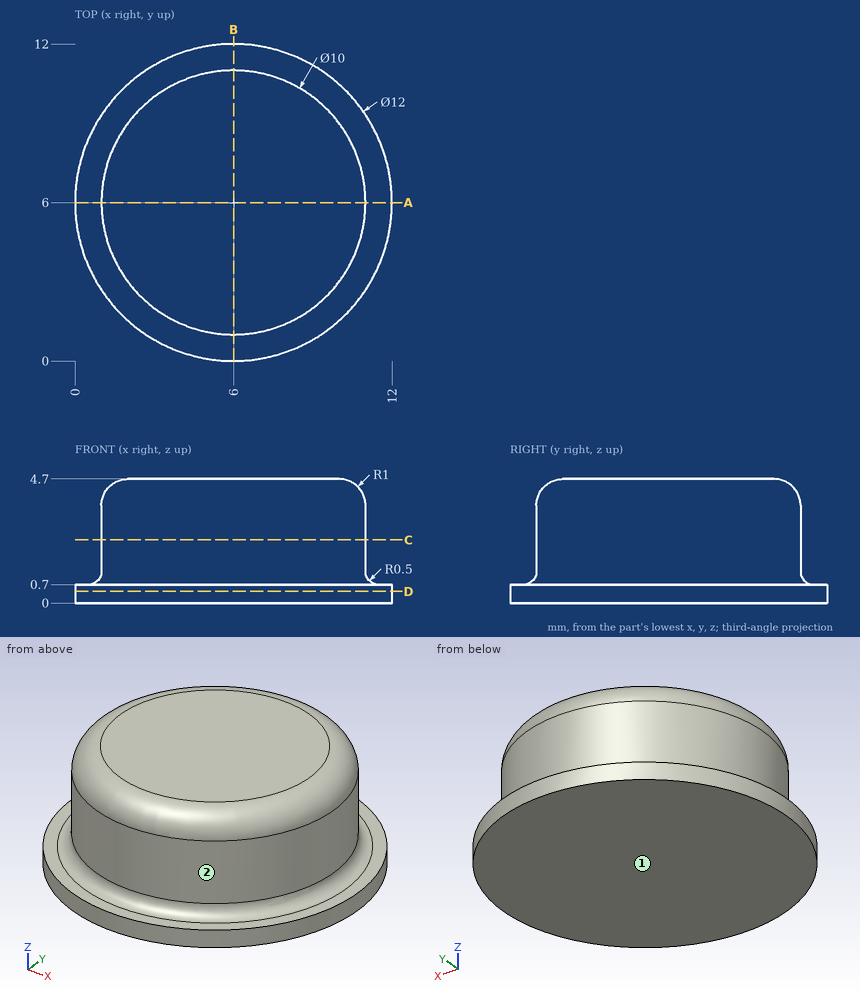
Source: three-view drawing plus pictorial views. Frame: mm from the lowest corner of the part. A direction names the side the tool comes from. Give positions to 0.01 mm unless a question says otherwise; leave off trailing zeros. Loops run counter-clockwise (first coordinate to the right, second up) from the corner with the lowest first, then second, coordinate; pieces in that order, holes last. Notation, with made-up numbers: (-19.75, 77) -> (6.25, 77) arc R17 cw to (6.25, 109) -> close; hole circle Ø10 at (77.25, -7.5). An arc over 180 degrees is marked (long way). Put each result on its own line as item: value. Start each with the question number.
1) Contact query for flat-ended pins moving along their axis: P1, Ø1, axis at x = 5.5, z = 4, coming from the -Y side; P2, Ø2, axis at x = 2, z = 2, coming from the +Y side. Output: stop coordinate, or through.
2) Cut plane A-A (y = 6). Return loops of the section in (x, z), then the cut area to 3 significant figures.
3) Reachability of the marked faces 1 and 2 from +Z, -Z, +X, -X, +Y, -Y: full face, straight path, thin tool, end or side. Return the list, or none.
4) Material intervals for probe 1 along Z at (x, y) = (10, 10.25); probe 2 along X at (y, z) = (3, 2.6); probe 3 along Y at (x, z) = (6, 2.05), sorted ascending.
5) Cut plane D-D (z = 0.45). Return loops of the section in (x, y), then the cut area to 3 significant figures.
6) Cut plane C-C (z = 2.4). Return loops of the section in (x, y), then the cut area to 3 significant figures.
Results are:
1. P1: stops at y = 1
1. P2: stops at y = 10
2. outline: (0, 0) -> (12, 0) -> (12, 0.7) -> (11.5, 0.7) arc R0.5 cw to (11, 1.2) -> (11, 3.7) arc R1 ccw to (10, 4.7) -> (2, 4.7) arc R1 ccw to (1, 3.7) -> (1, 1.2) arc R0.5 cw to (0.5, 0.7) -> (0, 0.7) -> close
2. area: 48.1 mm2
3. face 1: -Z, +X, -X, +Y, -Y
3. face 2: +Z
4. probe 1: z = 0 to 0.7
4. probe 2: x = 2 to 10
4. probe 3: y = 1 to 11
5. outline: circle Ø12 at (6, 6)
5. area: 113 mm2
6. outline: circle Ø10 at (6, 6)
6. area: 78.5 mm2
